Autodesk Inventor part; units mm, degrees
ref_plane "Arbeitsebene1" through (-114.5712, 43.4093, 38.3) normal (0, 0, -1) x (0, 1, 0)
ref_plane "YZ Plane" through (0, 0, 0) normal (1, 0, 0) x (0, 1, 0)
ref_plane "XZ Plane" through (0, 0, 0) normal (0, 1, 0) x (-1, 0, 0)
sketch "Skizze1" plane through (0, 0, 0) normal (0, 0, 1) x (1, 0, 0)
  line L0 (105.8135, 54.6424) -> (-70.1865, 54.6424) construction
  line L1 (-70.1865, 54.6424) -> (-70.1865, -55.3576) construction
  line L2 (-70.1865, -55.3576) -> (-86.1865, -55.3576) construction
  line L3 (-86.1865, -55.3576) -> (-86.1865, -56.6576) construction
  line L4 (112.8344, -56.6576) -> (-86.1865, -56.6576) construction
  line L5 (112.8344, -55.3576) -> (112.8344, -56.6576) construction
  line L6 (112.8344, -55.3576) -> (105.8135, -55.3576) construction
  line L7 (105.8135, -55.3576) -> (105.8135, 54.6424) construction
  line L8 (-104.5712, -45.4245) -> (-104.5712, -55.4245) construction
  line L9 (112.8135, -55.4245) -> (-104.5712, -55.4245) construction
  line L10 (112.8135, 46.962) -> (112.8135, -55.4245) construction
  line L11 (110.3928, 46.962) -> (112.8135, 46.962) construction
  arc A0 (110.3928, 50.262) -> (110.3928, 46.962) centre (110.3928, 48.612) ccw construction
  line L12 (112.8135, 50.262) -> (110.3928, 50.262) construction
  line L13 (112.8135, 54.6424) -> (112.8135, 50.262) construction
  line L14 (-86.7728, 54.6424) -> (112.8135, 54.6424) construction
  line L15 (-86.7728, 54.6424) -> (-86.7728, 44.6424) construction
  line L16 (-86.7728, 44.6424) -> (-96.7728, 44.6424) construction
  line L17 (-96.7728, 44.6424) -> (-96.7728, 54.6424) construction
  line L18 (-112.5712, 54.6424) -> (-96.7728, 54.6424) construction
  arc A1 (-112.5712, 54.6424) -> (-114.5712, 52.6424) centre (-112.5712, 52.6424) ccw construction
  line L19 (-114.5712, 44.6424) -> (-114.5712, 52.6424) construction
  line L20 (-114.5712, 44.6424) -> (-104.5712, 44.6424) construction
  line L21 (-104.5712, 44.6424) -> (-104.5712, 24.6424) construction
  line L22 (-104.5712, 24.6424) -> (-114.5712, 24.6424) construction
  line L23 (-114.5712, -45.4245) -> (-114.5712, 24.6424) construction
  line L24 (-114.5712, -45.4245) -> (-104.5712, -45.4245) construction
  circle A2 centre (-81.2226, -51.7118) radius 2 construction
  circle A3 centre (-109.5712, -50.4245) radius 1.75 construction
  arc A4 (-114.5712, -53.4245) -> (-112.5712, -55.4245) centre (-112.5712, -53.4245) ccw construction
  line L25 (-112.5712, -55.4245) -> (-104.5712, -55.4245) construction
  line L26 (-104.5712, -55.4245) -> (-104.5712, -45.4245) construction
  line L27 (-104.5712, -45.4245) -> (-114.5712, -45.4245) construction
  line L28 (-114.5712, -45.4245) -> (-114.5712, -53.4245) construction
  circle A5 centre (-91.7728, 49.6424) radius 1.75 construction
  line L29 (-86.7728, 54.6424) -> (-96.7728, 54.6424) construction
  line L30 (-96.7728, 54.6424) -> (-96.7728, 44.6424) construction
  line L31 (-96.7728, 44.6424) -> (-86.7728, 44.6424) construction
  line L32 (-86.7728, 44.6424) -> (-86.7728, 54.6424) construction
  line L33 (-114.5712, 42.6424) -> (-114.5712, 26.6424) construction
  arc A6 (-114.5712, 26.6424) -> (-112.5712, 24.6424) centre (-112.5712, 26.6424) ccw construction
  arc A7 (-112.5712, 44.6424) -> (-114.5712, 42.6424) centre (-112.5712, 42.6424) ccw construction
  line L34 (-114.5712, -56.6576) -> (-67.0712, -56.6576)
  line L35 (-67.0712, -56.6576) -> (-67.0712, 54.6424)
  line L36 (-67.0712, 54.6424) -> (-114.5712, 54.6424)
  line L37 (-114.5712, 54.6424) -> (-114.5712, -56.6576)
  point P0 (0, 0)
extrude "Extrusion1" add sketch "Skizze1" along normal blind 3
sketch "Skizze2" plane through (0, 0, 0) normal (0, 0, -1) x (-1, 0, 0)
  line L0 (104.5712, 43.4093) -> (114.5712, 43.4093)
  line L1 (104.5712, 53.4093) -> (104.5712, 43.4093)
  line L2 (112.5712, 53.4093) -> (104.5712, 53.4093)
  circle A0 centre (109.5712, 48.4093) radius 1.75
  line L3 (114.5712, 54.6424) -> (114.5712, -56.6576)
  circle A1 centre (91.7728, -51.6576) radius 1.75
  line L4 (86.7728, -46.6576) -> (86.7728, -56.6576)
  line L5 (114.5712, -56.6576) -> (67.0712, -56.6576)
  line L6 (96.7728, -46.6576) -> (86.7728, -46.6576)
  line L7 (96.7728, -56.6576) -> (96.7728, -46.6576)
  line L8 (114.5712, 54.6424) -> (114.5712, -56.6576)
  line L9 (104.5712, 43.4093) -> (114.5712, 43.4093)
  line L10 (114.5712, 43.4093) -> (114.5712, 53.4093)
  line L11 (114.5712, 53.4093) -> (104.5712, 53.4093)
  line L12 (104.5712, 53.4093) -> (104.5712, 43.4093)
  line L13 (86.7728, -56.6576) -> (96.7728, -56.6576)
  line L14 (96.7728, -56.6576) -> (96.7728, -46.6576)
  line L15 (96.7728, -46.6576) -> (86.7728, -46.6576)
  line L16 (86.7728, -46.6576) -> (86.7728, -56.6576)
  circle A2 centre (91.7728, -51.6576) radius 2.1
  circle A3 centre (109.5712, 48.4093) radius 2.1
  point P0 (0, 0)
  dimension "d3" = 4.2
  dimension "d4" = 4.2
ref_plane "Arbeitsebene1" through (-114.5712, 43.4093, 38.3) normal (0, 0, -1) x (0, 1, 0)
extrude "Extrusion2" add sketch "Skizze2" against normal up to surface (38.3 mm away) contours L1 L2 L11 L3 L0 | L5 L4 L6 L7
sketch "Skizze3" plane through (0, 0, 0) normal (0, 0, -1) x (-1, 0, 0)
  circle A0 centre (91.7728, -51.6576) radius 2.1
  circle A1 centre (109.5712, 48.4093) radius 2.1
  point P0 (0, 0)
hole "Bohrung1" at (-109.5712, 48.4093, 0) at (-91.7728, -51.6576, 0) direction (0, 0, 1) diameter 4.2 depth 38.3 counterbore diameter 8 counterbore depth 25
fillet "Rundung1" radius 1 2 edges at (-91.7728, -55.6576, 0) (-109.5712, 44.4093, 0)
sketch "Skizze4" plane through (-114.5712, 54.6424, 0) normal (-1, 0, 0) x (0, 0, 1)
  line L0 (3, 0) -> (3, -1.2331) construction
  line L1 (0, 0) -> (3, 0) construction
  line L2 (0, 0) -> (0, -6.2331) construction
  line L3 (0, -6.2331) -> (0, -111.3) construction
  line L4 (0, -111.3) -> (3, -111.3) construction
  line L5 (3, -11.2331) -> (3, -111.3) construction
  line L6 (3, -11.2331) -> (38.3, -11.2331) construction
  line L7 (38.3, -1.2331) -> (38.3, -11.2331) construction
  line L8 (3, -1.2331) -> (38.3, -1.2331) construction
  line L9 (25, -102.3) -> (1, -102.3) construction
  line L10 (3, -111.3) -> (38.3, -111.3) construction
  line L11 (55.8, -3.2331) -> (55.8, -109.3) construction
  line L12 (0, -111.3) -> (55.8, -111.3)
  line L13 (55.8, -111.3) -> (55.8, 0)
  line L14 (55.8, 0) -> (0, 0)
  line L15 (0, 0) -> (0, -111.3)
  point P0 (0, -54.6424)
extrude "Extrusion4" add sketch "Skizze4" along normal blind 3
sketch "Skizze5" plane through (-67.0712, 54.6424, 3) normal (0, 1, 0) x (1, 0, 0)
  line L0 (0, 3) -> (-50.5, 3) construction
  line L1 (-50.5, -52.8) -> (-50.5, 3) construction
  line L2 (179.8847, -52.8) -> (-45.5, -52.8) construction
  line L3 (-50.5, 3) -> (0, 3)
  line L4 (0, 3) -> (0, -52.8)
  line L5 (0, -52.8) -> (-50.5, -52.8)
  line L6 (-50.5, -52.8) -> (-50.5, 3)
  point P0 (67.0712, 3)
extrude "Extrusion5" add sketch "Skizze5" along normal blind 3
fillet "Rundung2" radius 2 1 edges at (-117.5712, 57.6424, 27.9)
sketch "Skizze6" plane through (-67.0712, -56.6576, 0) normal (0, -1, 0) x (1, 0, 0)
  line L0 (-47.5, 3) -> (-29.7016, 3) construction
  line L1 (-47.5, 3) -> (-47.5, 55.8) construction
  line L2 (-47.5, 55.8) -> (-50.5, 55.8) construction
  line L3 (-50.5, 0) -> (-50.5, 55.8) construction
  line L4 (-50.5, 0) -> (-24.7016, 0) construction
  line L5 (-24.7016, 0) -> (0, 0) construction
  line L6 (0, 0) -> (0, 3) construction
  line L7 (-19.7016, 3) -> (0, 3) construction
  line L8 (-19.7016, 3) -> (-19.7016, 38.3) construction
  line L9 (-29.7016, 38.3) -> (-19.7016, 38.3) construction
  line L10 (-29.7016, 3) -> (-29.7016, 38.3) construction
  line L11 (0, 3) -> (0, 55.8) construction
  line L12 (-45.5, 55.8) -> (179.8847, 55.8) construction
  line L13 (-50.5, 55.8) -> (-48.5, 55.8)
  line L14 (0, 0) -> (-50.5, 0)
  line L15 (-50.5, 0) -> (-50.5, 55.8)
  line L16 (-50.5, 55.8) -> (0, 55.8)
  line L17 (0, 55.8) -> (0, 0)
  point P0 (67.0712, 0)
extrude "Extrusion6" add sketch "Skizze6" along normal blind 3
fillet "Rundung3" radius 2 3 edges at (-92.3212, -59.6576, 0) (-117.5712, -59.6576, 27.9) (-91.3212, 57.6424, 0)
sketch "Skizze7" plane through (0, 0, 3) normal (0, 0, 1) x (1, 0, 0)
  arc A0 (-117.5712, -57.6576) -> (-115.5712, -59.6576) centre (-115.5712, -57.6576) ccw construction
  line L0 (-67.0712, -59.6576) -> (-115.5712, -59.6576) construction
  line L1 (-67.0712, -56.6576) -> (-67.0712, -59.6576) construction
  line L2 (-67.0712, -56.6576) -> (-114.5712, -56.6576) construction
  line L3 (-114.5712, -56.6576) -> (-114.5712, 54.6424) construction
  line L4 (-67.0712, 54.6424) -> (-114.5712, 54.6424) construction
  line L5 (-67.0712, 54.6424) -> (-67.0712, 57.6424) construction
  line L6 (-115.5712, 57.6424) -> (-67.0712, 57.6424) construction
  arc A1 (-115.5712, 57.6424) -> (-117.5712, 55.6424) centre (-115.5712, 55.6424) ccw construction
  line L7 (-117.5712, 55.6424) -> (-117.5712, -57.6576) construction
  line L8 (112.8135, 53.4093) -> (-112.5712, 53.4093) construction
  line L9 (-67.0712, 54.6424) -> (-114.5712, 54.6424) construction
  line L10 (-67.0712, 55.6424) -> (-115.5712, 55.6424)
  line L11 (-67.0712, 54.6424) -> (-114.5712, 54.6424)
  line L12 (-114.5712, 54.6424) -> (-114.5712, 55.6424)
  line L13 (-114.5712, 55.6424) -> (-67.0712, 55.6424)
  line L14 (-67.0712, 55.6424) -> (-67.0712, 54.6424)
  point P0 (0, 0)
extrude "Extrusion7" cut sketch "Skizze7" along normal up to surface (52.8 mm away)
sketch "Skizze9" plane through (-117.5712, 54.6424, 0) normal (-1, 0, 0) x (0, 0, 1)
  line L0 (2, -112.3) -> (2, 1) construction
  line L1 (55.8, -112.3) -> (2, -112.3) construction
  line L2 (55.8, 1) -> (55.8, -112.3) construction
  line L3 (2, 1) -> (55.8, 1) construction
  line L4 (52.8, -101.3) -> (38.3, -101.3) construction
  line L5 (52.8, -81.3) -> (38.3, -81.3) construction
  line L6 (36.3, -99.3) -> (36.3, -83.3) construction
  line L7 (55.8, -111.3) -> (55.8, 1) construction
  line L8 (55.8, -101.3) -> (50.8, -101.3)
  line L9 (50.8, -77.9589) -> (50.8, -2.6275)
  line L10 (50.8, -2.6275) -> (55.8, -2.6275)
  line L11 (50.8, -101.3) -> (40.8, -101.3)
  line L12 (40.8, -101.3) -> (40.8, -81.3)
  line L13 (40.8, -81.3) -> (50.8, -81.3)
  line L14 (50.8, -81.3) -> (55.8, -81.3)
  line L15 (55.8, -77.9589) -> (50.8, -77.9589)
  line L16 (55.8, -2.6275) -> (55.8, -77.9589)
  line L17 (55.8, -81.3) -> (55.8, -101.3)
  point P0 (0, -54.6424)
  dimension "d31" = 5
extrude "Extrusion9" cut sketch "Skizze9" against normal blind 3
fillet "Rundung4" radius 1 8 edges at (-117.5712, -46.6576, 48.3) (-117.5712, -36.6576, 40.8) (-114.5712, -46.6576, 48.3) (-117.5712, -23.3164, 53.3) (-117.5712, -26.6576, 48.3) (-117.5712, 14.3492, 50.8) (-114.5712, 14.3492, 50.8) (-117.5712, 52.0149, 53.3)
sketch "Skizze10" plane through (-117.5712, 54.6424, 0) normal (-1, 0, 0) x (0, 0, 1)
  line L0 (38.3, -3.2331) -> (55.8, -3.2331) construction
  line L1 (38.3, -11.2331) -> (38.3, -3.2331) construction
  line L2 (52.8, -11.2331) -> (38.3, -11.2331) construction
  line L3 (52.8, -11.2331) -> (52.8, -81.3) construction
  line L4 (52.8, -81.3) -> (38.3, -81.3) construction
  line L5 (38.3, -87.2689) -> (38.3, -81.3) construction
  arc A0 (38.3, -87.2689) -> (39.4111, -89.0605) centre (40.3, -87.2689) ccw construction
  arc A1 (40.7863, -91.0383) -> (39.4111, -89.0605) centre (38.3, -91.3) ccw construction
  line L6 (40.4663, -91.0383) -> (40.7863, -91.0383) construction
  line L7 (40.4663, -91.0383) -> (40.4663, -91.5741) construction
  line L8 (40.4663, -91.5741) -> (40.7849, -91.5741) construction
  arc A2 (39.4111, -93.5395) -> (40.7849, -91.5741) centre (38.3, -91.3) ccw construction
  arc A3 (39.4111, -93.5395) -> (38.3, -95.3311) centre (40.3, -95.3311) ccw construction
  line L9 (38.3, -101.3) -> (38.3, -95.3311) construction
  line L10 (52.8, -101.3) -> (38.3, -101.3) construction
  line L11 (52.8, -101.3) -> (52.8, -109.3) construction
  line L12 (55.8, -109.3) -> (52.8, -109.3) construction
  line L13 (55.8, -3.2331) -> (55.8, -109.3) construction
  arc A4 (40.8, -83.9404) -> (40.8, -98.6596) centre (38.3, -91.3) ccw
  line L14 (40.8, -101.3) -> (40.8, -81.3)
  line L15 (40.8, -98.6596) -> (40.8, -83.9404)
  point P0 (0, -54.6424)
extrude "Extrusion10" cut sketch "Skizze10" against normal blind 3
fillet "Rundung5" radius 1 6 edges at (-114.5712, -36.6576, 30.5274) (-117.2456, -29.2142, 40.5383) (-117.2456, -44.1009, 40.5383) (-115.5712, -29.298, 40.8) (-115.5712, -44.0172, 40.8) (-117.5712, -36.6576, 30.5274)
properties part number "PowerS_cap"
Check sheet for the modelled part. Datum: model origin and axes. Units: mm. A direction names the side the tool comes from. Give positions to 0.01 mm unless a question says otherwise; leave off trailing zeros. Order: outer loops, then holes, each group sorted by start corner. A loop starts at its lowest first (then second) coordinate and runs counter-clockwise, first axis right, second up. Notation, with made-up numbers: (21, 20.5) -> (74, 20.5) arc R22 cw to (74, 49.5) -> close; hole circle Ø10 at (34, 25.25). An arc over 180 degrees is marked (long way). Use CSV: the item, a comma, the result in double quotes. Start each with the question number.
1) Set-up check for faces 4 (the face through (-87.868, -52.525, 13.168)), 5 (the face through (-86, -56.658, 30)), 6 (the face through (-110, 53.409, 20)): record each of +Z, -Z, +X, -X, +Y, -Y from which the full face is reachable in a straight line by a thin tool's end or side.
2) Sectioned sample at B-B, the plane y = 10.5. Record the boundary of the cut face in (x, z).
3) Mould release check, pull along Z, two halves, no side actions. Record for faces 1 (the face through (-116.08, -36.47, 30.53)), 2 (the face through (-91, 0, 3)), 3 (the face through (-86.773, -52, 20)): released by +Z, released by -Z, zero draft, split by the parting line, or undercut.
4) Material ranges on line 1 (X direction, y = -51.5, z = 13); line 2 (Y direction, x = -93.5, z = 19.5); line 3 (Y direction, x = -79, z = 18.5), recorded low to high. Write a range as from..to.
5) Sectioned sample at A-A, the plane z = 48.5. Record the boundary of the cut face in (x, y), plus the area to 3 significant figures.
6) Sectioned sample at C-C, the plane x = -78.5. Record the boundary of the cut face in (y, z), plus the area to 3 significant figures.
7) Go/stop test with flat-tipped pins: P1, Ø11, axis at x = -90.5, y = -49.5, coming from the +Z side; P2, Ø1, axis at y = -13.5, z = 41.5, coming from the +X side; P3, Ø1.5, axis at x = -89.5, y = -20.5, coming from the +Z side. Record where each tip stops, or that it passes through.
8) Sectioned sample at D-D, the plane z = 33. Give the number of separate pieces and of enclosed holes in the cut face, plus the area to 3 significant figures.
Recorded:
1,face 4,"-Z"
1,face 5,"+Z"
1,face 6,"+Z, +X"
2,outline,"(-117.57, 2) arc R2 ccw to (-115.57, 0) -> (-67.07, 0) -> (-67.07, 3) -> (-114.57, 3) -> (-114.57, 49.8) arc R1 ccw to (-115.57, 50.8) -> (-116.57, 50.8) arc R1 ccw to (-117.57, 49.8) -> close"
3,face 1,"undercut"
3,face 2,"released by +Z"
3,face 3,"zero draft"
4,line 1,"-117.57..-114.57, -96.77..-95.77, -87.78..-86.77"
4,line 2,"-59.66..-55.27, -48.05..-46.66, 55.64..57.64"
4,line 3,"-59.66..-56.66, 55.64..57.64"
5,outline,"(-117.57, -57.66) arc R2 ccw to (-115.57, -59.66) -> (-67.07, -59.66) -> (-67.07, -56.66) -> (-114.57, -56.66) -> (-114.57, -47.66) arc R1 ccw to (-115.57, -46.66) -> (-116.57, -46.66) arc R1 ccw to (-117.57, -47.66) -> close; (-117.57, -25.66) arc R1 ccw to (-116.57, -26.66) -> (-114.57, -26.66) -> (-114.57, 55.64) -> (-67.07, 55.64) -> (-67.07, 57.64) -> (-115.57, 57.64) arc R2 ccw to (-117.57, 55.64) -> close"
5,area,"527 mm2"
6,outline,"(-59.66, 2) arc R2 ccw to (-57.66, 0) -> (55.64, 0) arc R2 ccw to (57.64, 2) -> (57.64, 55.8) -> (55.64, 55.8) -> (55.64, 3) -> (-56.66, 3) -> (-56.66, 55.8) -> (-59.66, 55.8) -> close"
6,area,"614 mm2"
7,P1,"z = 38.3"
7,P2,"x = -114.57"
7,P3,"z = 3"
8,separate pieces,"2"
8,enclosed holes,"2"
8,area,"725 mm2"
